from build123d import *

# Parameters (mm, degrees)
F0_W      = 25.4
F0_H      = 25.4
F1_DEPTH  = 12.7
F6_R      = 2.366031
F6_R_2    = 2.397035
F6_R_3    = 2.418186
F6_R_4    = 2.249071
F6_R_5    = 2.3495
F8_DEPTH  = 0.508
F3_R      = 2.3495
F9_DEPTH  = 0.508
F4_R      = 2.3495
F10_DEPTH = 0.508
F5_R      = 2.3495
F11_DEPTH = 0.508
F7_R      = 2.3495
F7_R_2    = 2.451766
F12_DEPTH = 0.508
F2_R      = 2.355595
F2_R_2    = 2.347424
F2_R_3    = 2.3495
F13_DEPTH = 0.508
F14_DEPTH = 0.508
F15_R     = 1.27


with BuildPart() as f1:
    # F0 (on Top) → F1 (new body, symmetric)
    with BuildSketch(Plane.XY):
        Rectangle(F0_W, F0_H)
    extrude(amount=F1_DEPTH, both=True)

    # F6 (on face) → F8 (join)
    with BuildSketch(Plane.YZ.offset(12.7)):
        with Locations((6.863432, 7.388731)):
            Circle(F6_R)
        with Locations((7.110631, -7.731593)):
            Circle(F6_R_2)
        with Locations((-6.361702, -7.607994)):
            Circle(F6_R_3)
        Circle(F6_R_4)
        with Locations((-7.638895, 8.006728)):
            Circle(F6_R_5)
    extrude(amount=F8_DEPTH)

    # F3 (on face) → F9 (join)
    with BuildSketch(Plane.XY.offset(12.7)):
        Circle(F3_R)
    extrude(amount=F9_DEPTH)

    # F4 (on face) → F10 (join)
    with BuildSketch(Plane(origin=(0, 12.7, 0), x_dir=(-1, 0, 0), z_dir=(0, 1, 0))):
        with Locations((-6.917292, 6.473729)):
            Circle(F4_R)
        with Locations((6.729059, 6.646467)):
            Circle(F4_R)
        with Locations((6.556321, -6.308929)):
            Circle(F4_R)
        with Locations((-6.053598, -6.481668)):
            Circle(F4_R)
    extrude(amount=F10_DEPTH)

    # F5 (on face) → F11 (join)
    with BuildSketch(Plane.XZ.offset(12.7)):
        with Locations((6.381141, 5.995322)):
            Circle(F5_R)
    extrude(amount=-F11_DEPTH)

    # F7 (on face) → F12 (join)
    with BuildSketch(Plane(origin=(-12.7, 0, 0), x_dir=(0, -1, 0), z_dir=(-1, 0, 0))):
        with Locations((-6.925553, 8.001271)):
            Circle(F7_R)
        with Locations((-6.925553, 0)):
            Circle(F7_R)
        with Locations((-6.925553, -7.923216)):
            Circle(F7_R)
        with Locations((8.158201, 8.001271)):
            Circle(F7_R)
        with Locations((8.158201, 0)):
            Circle(F7_R_2)
        with Locations((8.257111, -7.923216)):
            Circle(F7_R)
    extrude(amount=F12_DEPTH)

    # F2 (on face) → F13 (join)
    with BuildSketch(Plane(origin=(0, 0, -12.7), x_dir=(1, 0, 0), z_dir=(0, 0, -1))):
        Circle(F2_R)
        with Locations((-6.368103, -6.368103)):
            Circle(F2_R_2)
        with Locations((7.108342, 6.695065)):
            Circle(F2_R_3)
    extrude(amount=F13_DEPTH)

    # F5 (on face) → F14 (join)
    with BuildSketch(Plane.XZ.offset(12.7)):
        with Locations((-6.024025, -5.776247)):
            Circle(F5_R)
        with Locations((6.381141, 5.995322)):
            Circle(F5_R)
    extrude(amount=F14_DEPTH)

    # F15
    f15_edges = [f1.edges().sort_by_distance(p)[0] for p in [
        (12.7, 0, 12.7),
        (12.7, -12.7, 0),
        (0, -12.7, 12.7),
        (-12.7, -12.7, 0),
        (-12.7, 0, 12.7),
        (-12.7, 12.7, 0),
        (-12.7, 0, -12.7),
        (0, 12.7, 12.7),
        (12.7, 12.7, 0),
        (0, -12.7, -12.7),
        (12.7, 0, -12.7),
        (0, 12.7, -12.7),
    ]]
    fillet(f15_edges, radius=F15_R)


solid = f1.part
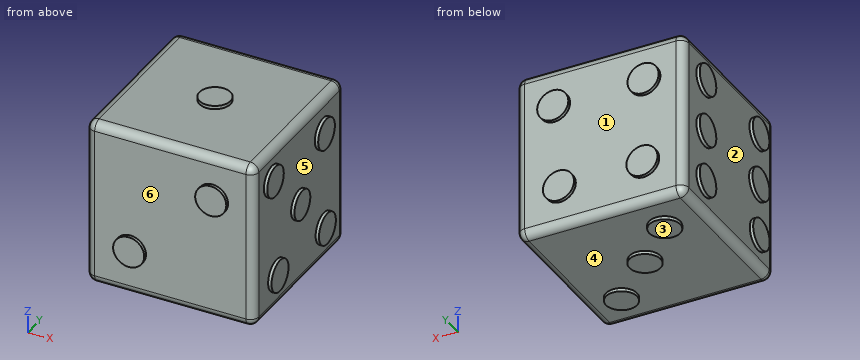
Input: part model. Units: mm. Frame: model coordinates. Face numbers are marked on the shaded views. A direction names the side the tool comes from. Give positions to 0.01 mm unless a question says otherwise; leave off trailing zeros. Order: outer loops, then holes, each group sorted by start corner. A loop starts at its lowest first (then second) coordinate and runs counter-clockwise, first axis right, second up.
Q1. Section D-D on x = 0. Output: boundary loops of the cut face in (y, z).
Checked values:
outline: (-12.7, -11.43) arc R1.27 ccw to (-11.43, -12.7) - (-2.36, -12.7) - (-2.36, -13.21) - (2.36, -13.21) - (2.36, -12.7) - (11.43, -12.7) arc R1.27 ccw to (12.7, -11.43) - (12.7, 11.43) arc R1.27 ccw to (11.43, 12.7) - (2.35, 12.7) - (2.35, 13.21) - (-2.35, 13.21) - (-2.35, 12.7) - (-11.43, 12.7) arc R1.27 ccw to (-12.7, 11.43) - close
Q2. Section B-B on z = 0. Output: boundary loops of the cut face in (x, y), and give its area (3 significant figures).
Checked values:
outline: (-13.21, -10.61) - (-12.7, -10.61) - (-12.7, -11.43) arc R1.27 ccw to (-11.43, -12.7) - (11.43, -12.7) arc R1.27 ccw to (12.7, -11.43) - (12.7, -2.25) - (13.21, -2.25) - (13.21, 2.25) - (12.7, 2.25) - (12.7, 11.43) arc R1.27 ccw to (11.43, 12.7) - (-11.43, 12.7) arc R1.27 ccw to (-12.7, 11.43) - (-12.7, 9.28) - (-13.21, 9.28) - (-13.21, 4.58) - (-12.7, 4.58) - (-12.7, -5.71) - (-13.21, -5.71) - close
area: 651 mm2
Q3. Section A-A on y = 0. Output: boundary loops of the cut face in (x, z).
Checked values:
outline: (-12.7, -11.43) arc R1.27 ccw to (-11.43, -12.7) - (-2.36, -12.7) - (-2.36, -13.21) - (2.36, -13.21) - (2.36, -12.7) - (11.43, -12.7) arc R1.27 ccw to (12.7, -11.43) - (12.7, -2.25) - (13.21, -2.25) - (13.21, 2.25) - (12.7, 2.25) - (12.7, 11.43) arc R1.27 ccw to (11.43, 12.7) - (2.35, 12.7) - (2.35, 13.21) - (-2.35, 13.21) - (-2.35, 12.7) - (-11.43, 12.7) arc R1.27 ccw to (-12.7, 11.43) - close
Q4. Section C-C on x = 11. Output: boundary loops of the cut face in (y, z).
Checked values:
outline: (-12.7, -11.43) arc R1.27 ccw to (-11.43, -12.7) - (11.43, -12.7) arc R1.27 ccw to (12.7, -11.43) - (12.7, 11.43) arc R1.27 ccw to (11.43, 12.7) - (-11.43, 12.7) arc R1.27 ccw to (-12.7, 11.43) - close
Q5. Contact query for flat-ended pins moving along their axis: pin 1 Ø10 at (x, y) = (3.5, 9) entering from +Z; pin 2 Ø3 at (x, z) = (3, -8) entering from -Y; pin 3 Ø6 at (y, z) = (-6.5, 3) entering from -X; pin 4 Ø3 at (x, y) = (-8, -4.5) entering from -Z. Output: stop coordinate, or through.
Checked values:
pin 1: stops at z = 12.7
pin 2: stops at y = -12.7
pin 3: stops at x = -13.21
pin 4: stops at z = -12.7
Q6. Ray query, probe 1 along X at (y, z) = (-2, -9.25). Return the intervals inside material, ascending.
Checked values:
probe 1: x = -12.7 to 12.7
Q7. Draft query along X for the marked faces 1, 2 and 3. Return one class per face: +X half, -X half, draft (parallel to the pull), parting line (faces both ways), or undercut.
Checked values:
face 1: undercut
face 2: -X half
face 3: draft
Q8. Set-up query: the marked faces 4, 5 and 6. Return all of +Z, -Z, +X, -X, +Y, -Y with unobstructed straight access to the full face (end or side cutting, diameter ignored); none if empty.
Checked values:
face 4: -Z
face 5: +X
face 6: -Y
